```python
from build123d import *

# Parameters (mm, degrees)
BOSS_EXTRUDE1_DEPTH = 3.175
SKETCH3_R           = 2.032
CUT_EXTRUDE1_DEPTH  = 129.616894788
FILLET1_R           = 3.175
FILLET2_R           = 101.6
FILLET3_R           = 6.35


with BuildPart() as part:
    # Sketch2 → Boss-Extrude1 (new body)
    with BuildSketch(Plane.XY):
        Polygon((120.65, -44.45), (120.65, 44.45), (114.870442245, 44.45), (0, 6.684375152), (-114.870442245, 44.45), (-120.65, 44.45), (-120.65, -44.45), (-114.870442245, -44.45), (0, -6.684375152), (114.870442245, -44.45), align=None)
        Polygon((-111.125, 29.849871423), (-20.331641088, 0), (-111.125, -29.849871423), align=None, mode=Mode.SUBTRACT)
        Polygon((20.331641088, 0), (111.125, -29.849871423), (111.125, 29.849871423), align=None, mode=Mode.SUBTRACT)
    extrude(amount=BOSS_EXTRUDE1_DEPTH)

    # Sketch3 → Cut-Extrude1 (cut, through all)
    with BuildSketch(Plane.XY.offset(3.175)):
        with Locations((-115.8875, 38.1)):
            Circle(SKETCH3_R)
        with Locations((-115.8875, -38.1)):
            Circle(SKETCH3_R)
        with Locations((115.8875, 38.1)):
            Circle(SKETCH3_R)
        with Locations((115.8875, -38.1)):
            Circle(SKETCH3_R)
    extrude(amount=-CUT_EXTRUDE1_DEPTH, mode=Mode.SUBTRACT)

    # Fillet1
    fillet1_edges = [part.edges().sort_by_distance(p)[0] for p in [
        (114.870442245, -44.45, 1.5875),
        (-114.870442245, -44.45, 1.5875),
        (-120.65, -44.45, 1.5875),
        (-120.65, 44.45, 1.5875),
        (-114.870442245, 44.45, 1.5875),
        (114.870442245, 44.45, 1.5875),
        (120.65, 44.45, 1.5875),
        (120.65, -44.45, 1.5875),
    ]]
    fillet(fillet1_edges, radius=FILLET1_R)

    # Fillet2
    fillet2_edges = [part.edges().sort_by_distance(p)[0] for p in [
        (0, -6.684375152, 1.5875),
        (0, 6.684375152, 1.5875),
    ]]
    fillet(fillet2_edges, radius=FILLET2_R)

    # Fillet3
    fillet3_edges = [part.edges().sort_by_distance(p)[0] for p in [
        (-111.125, -29.849871423, 1.5875),
        (-20.331641088, 0, 1.5875),
        (-111.125, 29.849871423, 1.5875),
        (111.125, -29.849871423, 1.5875),
        (111.125, 29.849871423, 1.5875),
        (20.331641088, 0, 1.5875),
    ]]
    fillet(fillet3_edges, radius=FILLET3_R)


solid = part.part
```
CAD build for the part. Positions are in the model's coordinates, mm. A direction names the side the tool comes from. Round coordinates to 2 decimals unless told otherwise and drop trailing zeros. Write each loop counter-clockwise with the first axis right and the second up, starting at its lowest first coordinate (ties: lowest second). Pieces come first, ordered by that corner, then holes. Notation, with made-up numbers: (52.5, -1.75) - (85.5, -1.75) arc R26 cw to (85.5, 27.25) - close; hole circle Ø1 at (17, -35.75). An arc over 180 degrees is marked (long way). Write item = value, one per line. Start each with the question number.
Q1. Band-saw the part on A-A (y = 0). Give the cut face in (x, z) (3 decimals), then the cut area to 3 significant figures.
Q2. Band-saw the part on B-B (x = 56.5). Give the cut face in (y, z) (3 decimals).
Q3. Which spindle directions (+Z, -Z, +X, -X, +Y, -Y) get a long thin tool onto all of the face, cutting with end or side? Do faces 1 (the flat face through (-73.638, -30.894, 1.565)), 2 (the flat face through (-1, 4, 3.175)), 3 (the flat face through (-71.185, 16.719, 1.565)), 4 (the flat face through (-72.481, 30.514, 1.565)). Say none if no direction does.
Q4. Band-saw the part on D-D (x = -20.5). Give the cut face in (y, z) (3 decimals).
Q5. Probe L1, parallel to X at y = -3, z = 1.75 (3 decimals); L2, parallel to X at y = -1, z = 2 (3 decimals); L3, parallel to Y at x = -3, z = 1.1. List the from-to ranges inside material, lowest first. Write a range as from..to.
Q6. Mould opens along X. For faces 5 (the cylindrical face through (-108.57, 26.17, 1.61)), 6 (the flat face through (-1, 4, 0)), 7 (the flat face through (73.638, 30.894, 1.565)) say: pulls with the +X half, pulls with the -X half, needs draft (parallel to the pull), parting line crosses it, or undercut.
Q7. Band-saw the part on C-C (z = 2). Count the separate pieces of the cut face and the enclosed holes in it, then the cut area to 3 significant figures.
Q8. Drop a flat-ended pin along its axis: pin 1 (1.5 mm diameter, centred on x = -72.5, z = 2.5, fed in from +Y). Give the stop position or say it passes through.
Answers below:
q1.outline = (-120.65, 0) - (-111.125, 0) - (-111.125, 3.175) - (-120.65, 3.175) - close; (-34.313, 0) - (34.313, 0) - (34.313, 3.175) - (-34.313, 3.175) - close; (111.125, 0) - (120.65, 0) - (120.65, 3.175) - (111.125, 3.175) - close
q1.area = 278 mm2
q2.outline = (-25.26, 0) - (-11.891, 0) - (-11.891, 3.175) - (-25.26, 3.175) - close; (11.891, 0) - (25.26, 0) - (25.26, 3.175) - (11.891, 3.175) - close
q3.face_1 = +Z, -Z, -Y
q3.face_2 = +Z, +X, -X, +Y, -Y
q3.face_3 = +Z, -Z
q3.face_4 = +Z, -Z, +Y
q4.outline = (-14.124, 0) - (14.124, 0) - (14.124, 3.175) - (-14.124, 3.175) - close
q5.L1 = -120.65..-111.125, -35.067..35.067, 111.125..120.65
q5.L2 = -120.65..-111.125, -34.393..34.393, 111.125..120.65
q5.L3 = -12.08..12.08
q6.face_5 = undercut
q6.face_6 = needs draft
q6.face_7 = undercut
q7.separate_pieces = 1
q7.enclosed_holes = 6
q7.area = 7,740 mm2
q8.pin_1 = 30.77
